Here's the drawing with two shaded views (mm, measured from the low corner). I have some questions. A direction names the side the tool comes from. Give positions to 0.01 mm unless a question says otherwise; leave off trailing zeros. Write each loop counter-clockwise with the first axis right and the second up, starting at its lowest first coordinate (ties: lowest second). Pieces come first, ordered by that corner, then holes.
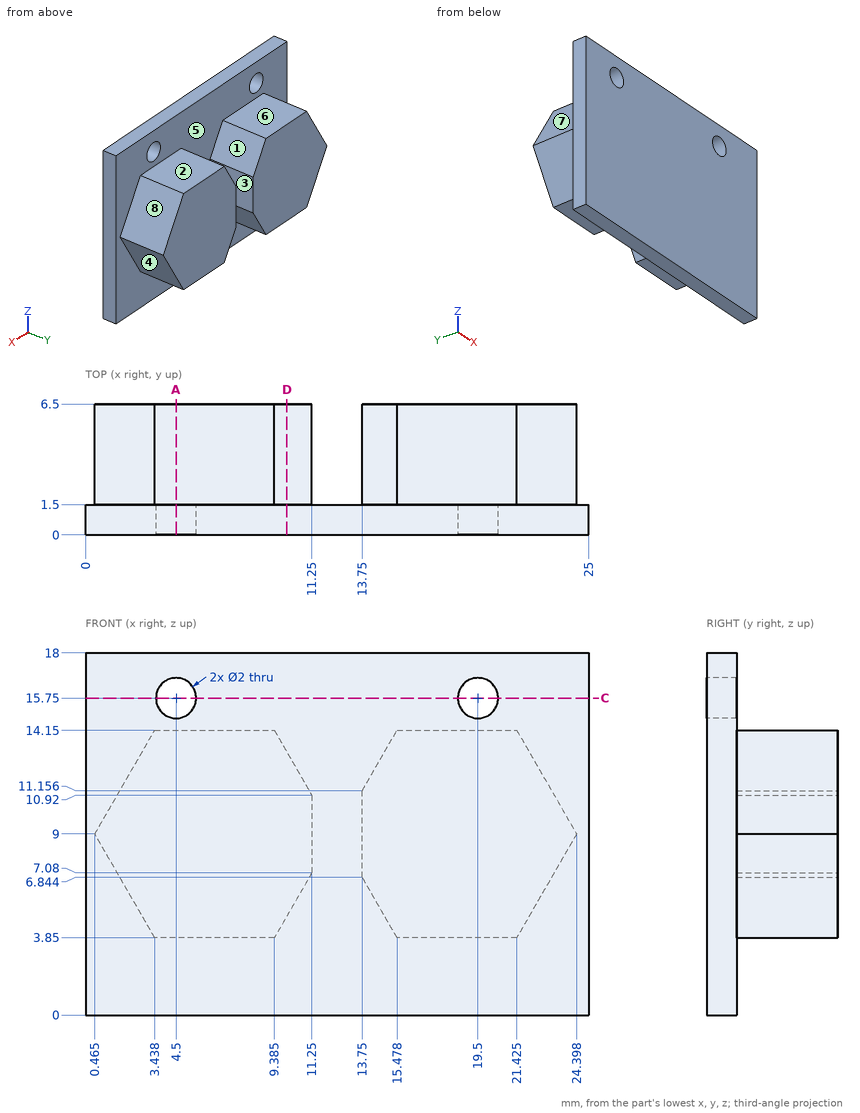
1) If we mould it in two halves opening along X, with no side actions, what happens to the marked faces 1, 2, 3 and 4? For each: +X half, -X half, draft (parallel to the pull), parting line (faces both ways), or undercut.
Values follow:
face 1: undercut
face 2: draft
face 3: undercut
face 4: +X half
2) Suppose I cut it at D-D on x = 10. Write out the boundary of the cut face in (y, z) (1 decimal).
Values follow:
outline: (0, 0) - (1.5, 0) - (1.5, 4.9) - (6.5, 4.9) - (6.5, 13.1) - (1.5, 13.1) - (1.5, 18) - (0, 18) - close
3) Please list where these lines run through material, in increasing order: L1, parallel to Z at x = 4.5, y = 0.5; L2, parallel to Y at x = 2.5, z = 12.75; L3, parallel to Z at x = 9.25, y = 3.25.
Values follow:
L1: z = 0 to 14.75, 16.75 to 18
L2: y = 0 to 1.5
L3: z = 3.85 to 14.15
4) Suppose I cut it at C-C on z = 15.75. Write out the boundary of the cut face in (x, y), plus the area to 3 significant figures.
Values follow:
outline: (0, 0) - (3.5, 0) - (3.5, 1.5) - (0, 1.5) - close; (5.5, 0) - (18.5, 0) - (18.5, 1.5) - (5.5, 1.5) - close; (20.5, 0) - (25, 0) - (25, 1.5) - (20.5, 1.5) - close
area: 31.5 mm2
5) For pin 1 Ø1.5 at (y, z) = (5.5, 11) entering from -X; pin 2 Ø2.5 at (x, z) = (19.5, 15.75) entering from +Y; pin 3 Ø3.5 at (y, z) = (3.5, 9) entering from -X (3 decimals), each with a flat end and sliding along its axis, tell me the tip position at first contact or that it passes through.
Values follow:
pin 1: stops at x = 1.19
pin 2: stops at y = 1.5
pin 3: stops at x = 0.465
6) Suppose I cut it at A-A on x = 4.5. Write out the boundary of the cut face in (y, z), plus the area to 3 significant figures.
Values follow:
outline: (0, 0) - (1.5, 0) - (1.5, 3.85) - (6.5, 3.85) - (6.5, 14.15) - (1.5, 14.15) - (1.5, 14.75) - (0, 14.75) - close; (0, 16.75) - (1.5, 16.75) - (1.5, 18) - (0, 18) - close
area: 75.5 mm2
7) For the marked faces 5, 6, 7 and 8, which set-ups out of +Z, -Z, +X, -X, +Y, -Y let a thin tool reach every point of the face, with its end or its side?
Values follow:
face 5: +Y
face 6: +Z, +X, -X, +Y
face 7: +Z, -X, +Y
face 8: +Z, +X, +Y
